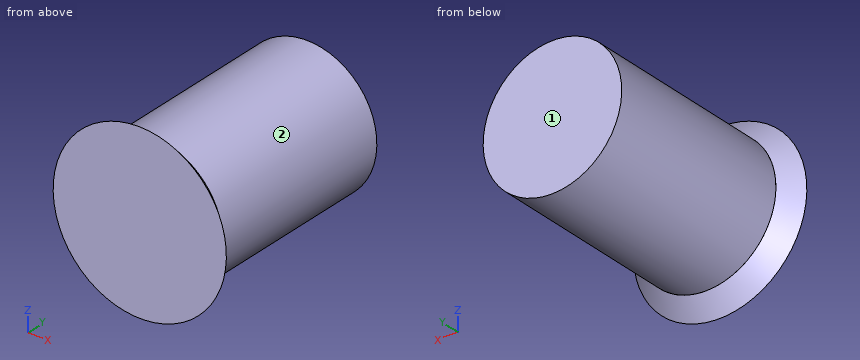
from build123d import *

# Parameters (mm, degrees)
ESQUISSE1_R        = 15
BOSS_EXTRU_1_DEPTH = 3
CHANFREIN1_SIZE    = 3
ESQUISSE2_R        = 12
BOSS_EXTRU_2_DEPTH = 34


with BuildPart() as part:
    # Esquisse1 → Boss.-Extru.1 (new body)
    with BuildSketch(Plane(origin=(0, 0, 0), x_dir=(1, 0, 0), z_dir=(0, 1, 0))):
        with Locations(Location((0, 0, 0), (0, 0, 270))):
            Circle(ESQUISSE1_R)
    extrude(amount=BOSS_EXTRU_1_DEPTH)

    # Chanfrein1
    chanfrein1_edges = [part.edges().sort_by_distance(p)[0] for p in [
        (0, 3, -15),
    ]]
    chamfer(chanfrein1_edges, length=CHANFREIN1_SIZE - 0.0001)  # a hair under: the kernel refuses the full size

    # Esquisse2 → Boss.-Extru.2 (add)
    with BuildSketch(Plane(origin=(0, 3, 0), x_dir=(1, 0, 0), z_dir=(0, 1, 0))):
        with Locations(Location((0, 0, 0), (0, 0, 90))):
            Circle(ESQUISSE2_R)
    extrude(amount=BOSS_EXTRU_2_DEPTH)


solid = part.part
Can you work these out from the model? Positions are in its coordinate system, mm. Face numbers are marked on the shaded views. A direction names the side the tool comes from. Give positions to 0.01 mm unless a question says otherwise; leave off trailing zeros. Order: outer loops, then holes, each group sorted by start corner. A loop starts at its lowest first (then second) coordinate and runs counter-clockwise, first axis right, second up. Notation, with made-up numbers: M -10.5,86 L 16.5,86 A18 ccw 16.5,99 Z; hole C -3.75,-15.5 d2. An arc over 180 degrees is marked long. Use a Markdown table: item, result. Add a question column.
Item 1: For the marked faces 1 and 2, which set-ups out of +Z, -Z, +X, -X, +Y, -Y let a thin tool reach every point of the face, with its end or its side?
Item 2: Suppose I cut it at C-C (y = 32.5). List the corners of the cut face in (x, z) for me, then the cut area to 3 significant figures.
Item 3: If I drill on L1, parallel to Z at x = -8.5, y = 12; L2, parallel to X at y = 20, z = -4.5; L3, parallel to Z at x = -3.75, y = 2, over which ranges is the centre line in solid material (lowest first)? Write a range as [from, to].
Item 4: Will these pins go through, and if not, where does the flat tip stop? pin 1 (5 mm diameter, centred on y = 21, z = -1, fed in from -X); pin 2 (4 mm diameter, centred on y = 27.5, z = 5, fed in from -X); pin 3 (2 mm diameter, centred on x = 8, y = 13, fed in from -Z).
Answer sheet:
| question | item | result |
|---|---|---|
| 1 | face 1 | +Z, -Z, +X, -X, +Y |
| 1 | face 2 | +Y |
| 2 | outline | C 0,0 d24 |
| 2 | area | 452 mm² |
| 3 | L1 | z = [-8.47, 8.47] |
| 3 | L2 | x = [-11.12, 11.12] |
| 3 | L3 | z = [-12.45, 12.45] |
| 4 | pin 1 | stops at x = -12 |
| 4 | pin 2 | stops at x = -11.62 |
| 4 | pin 3 | stops at z = -9.75 |
